Check sheet for the modelled part. Datum: model origin and axes. Units: mm. A direction names the side the tool comes from. Give positions to 0.01 mm unless a question says otherwise; leave off trailing zeros. Loops run counter-clockwise (first coordinate to the right, second up) from the corner with the lowest first, then second, coordinate; pieces in that order, holes last. Notation, with made-up numbers: (28.25, 76) - (76.25, 76) arc R30 ccw to (76.25, 108) - close; hole circle Ø2 at (-20, 7.25). An arc over 180 degrees is marked (long way). Answer in a Markdown table with one row per item. Add a question column.
(1) Sectioned sample at A-A on x = 5.5. Enter the section's corners in (y, z).
(2) Sectioned sample at B-B on y = 3. Enter the section's corners in (x, z).
(3) Sectioned sample at C-C on x = 13.5. Enter the section's corners in (y, z), then the cut area to 3 significant figures.
(4) Draft check along Z on faces 6 (the face through (5.57, 2.94, -4)), 7 (the face through (-5.5, 4.3, -4.6)), 8 (the face through (5.652, -0.74, -2.053)). Enter one of: released by +Z, released by -Z, zero draft, split by the parting line, or undercut.
(5) Sectioned sample at D-D on z = -10.25. Enter the section's corners in (x, y), then the cut area to 3 significant figures.
(6) Set-up check for faces 1 (the face through (5.4, 0, -1.9)), 2 (the face through (-6.355, 3.938, -7.763)), 3 (the face through (6.55, 6.74, -8.04)), 4 (the face through (17.345, 2.062, -7.763)), 5 (the face through (-2.7, 3.52, -4.2)): record each of +Z, -Z, +X, -X, +Y, -Y from which the full face is reachable in a straight line by a thin tool's end or side.
(7) Go/stop test with flat-tipped pins: P1, Ø3, axis at x = -4.5, y = 5.5, coming from the -Z side; P2, Ø4, axis at x = -1, y = 5.5, coming from the -Z side; P3, Ø2, axis at y = 5, z = -9.5, coming from the -X side. Record where each tip stops, or that it passes through.
(8) Thickness scan on L1, parallel to X at y = 1, z = -5.5; L2, parallel to X at y = 0.75, z = -5.5; L3, parallel to Y at x = 8, z = -3.25. Record the ranges inside material, lowest first.
from build123d import *

# Parameters (mm, degrees)
SKETCH1_W      = 11
SKETCH1_H      = 11
EXTRUDE1_DEPTH = 6
SKETCH2_R      = 1.4
EXTRUDE2_DEPTH = 5.5
EXTRUDE3_START = 5.5
SKETCH3_R      = 1.4
EXTRUDE3_DEPTH = 5.5
SKETCH4_R      = 2.75
EXTRUDE4_DEPTH = 1.5
SKETCH5_R      = 3.45
EXTRUDE5_DEPTH = 1.5
SKETCH6_R      = 2.45
EXTRUDE6_DEPTH = 1.7
EXTRUDE7_START = 1.7
SKETCH7_R      = 2.45
EXTRUDE7_DEPTH = 1.7
SKETCH8_R      = 1.5
EXTRUDE8_DEPTH = 24.091989953
FILLET1_R      = 5.5
FILLET3_R      = 0.5


with BuildPart() as part:
    # Sketch1 → Extrude1 (new body)
    with BuildSketch(Plane(origin=(0, 0, 0), x_dir=(1, 0, 0), z_dir=(0, 1, 0))):
        with Locations((5.5, 5.5)):
            Rectangle(SKETCH1_W, SKETCH1_H)
    extrude(amount=EXTRUDE1_DEPTH)

    # Sketch2 → Extrude2 (add)
    with BuildSketch(Plane(origin=(11, 0, 0), x_dir=(0, 0, -1), z_dir=(1, 0, 0))):
        with Locations(Location((5.5, 3, 0), (0, 0, 180))):
            Circle(SKETCH2_R)
    extrude(amount=EXTRUDE2_DEPTH)

    # Sketch3 → Extrude3 (add)
    with BuildSketch(Plane.ZY.offset(EXTRUDE3_START)):
        with Locations((-5.5, 3)):
            Circle(SKETCH3_R)
    extrude(amount=-EXTRUDE3_DEPTH)

    # Sketch4 → Extrude4 (add)
    with BuildSketch(Plane(origin=(0, 6, 0), x_dir=(1, 0, 0), z_dir=(0, 1, 0))):
        with Locations(Location((5.5, 5.5, 0), (0, 0, 90))):
            Circle(SKETCH4_R)
    extrude(amount=EXTRUDE4_DEPTH)

    # Sketch5 → Extrude5 (add)
    with BuildSketch(Plane.XZ):
        with Locations(Location((5.5, -5.5, 0), (0, 0, 270))):
            Circle(SKETCH5_R)
    extrude(amount=EXTRUDE5_DEPTH)

    # Sketch6 → Extrude6 (add)
    with BuildSketch(Plane(origin=(16.5, 0, 0), x_dir=(0, 0, -1), z_dir=(1, 0, 0))):
        with Locations((5.5, 3)):
            Circle(SKETCH6_R)
    extrude(amount=EXTRUDE6_DEPTH)

    # Sketch7 → Extrude7 (add)
    with BuildSketch(Plane.ZY.offset(5.5).offset(EXTRUDE7_START)):
        with Locations(Location((-5.5, 3, 0), (0, 0, 180))):
            Circle(SKETCH7_R)
    extrude(amount=-EXTRUDE7_DEPTH)

    # Sketch8 → Extrude8 (cut, through all)
    with BuildSketch(Plane.XZ.offset(1.5)):
        with Locations(Location((5.5, -5.5, 0), (0, 0, 270))):
            Circle(SKETCH8_R)
    extrude(amount=-EXTRUDE8_DEPTH, mode=Mode.SUBTRACT)

    # Fillet1
    # the kernel refuses this fillet: 5.5 mm, written as the material it takes off along each edge
    with BuildSketch(Plane(origin=(0, -13.75, 0), x_dir=(0, 0, -1), z_dir=(0, 1, 0))) as fillet1_piece_1_section:
        with BuildLine():
            CenterArc((FILLET1_R, -FILLET1_R), FILLET1_R, 90, 90)
            Line((0, -FILLET1_R), (0, 0))
            Line((0, 0), (FILLET1_R, 0))
        make_face()
    fillet1_piece_1 = extrude(amount=33.5, mode=Mode.PRIVATE)
    fillet1_piece_1 = fillet1_piece_1 - Plane(origin=(1.247523626, 3, -5.5), x_dir=(0, 0, 1), z_dir=(-1, 0, 0)) * Cylinder(1.4, 89, mode=Mode.PRIVATE)
    with BuildSketch(Plane(origin=(0, -13.75, -11), x_dir=(0, 0, 1), z_dir=(0, 1, 0))) as fillet1_piece_2_section:
        with BuildLine():
            CenterArc((FILLET1_R, FILLET1_R), FILLET1_R, 180, 90)
            Line((0, FILLET1_R), (0, 0))
            Line((0, 0), (FILLET1_R, 0))
        make_face()
    fillet1_piece_2 = extrude(amount=33.5, mode=Mode.PRIVATE)
    fillet1_piece_2 = fillet1_piece_2 - Plane(origin=(1.247523509, 3, -5.5), x_dir=(0, 0, 1), z_dir=(-1, 0, 0)) * Cylinder(1.4, 89, mode=Mode.PRIVATE)
    with BuildSketch(Plane(origin=(11, -13.75, -11), x_dir=(-1, 0, 0), z_dir=(0, 1, 0))) as fillet1_piece_3_section:
        with BuildLine():
            CenterArc((FILLET1_R, FILLET1_R), FILLET1_R, 180, 90)
            Line((0, FILLET1_R), (0, 0))
            Line((0, 0), (FILLET1_R, 0))
        make_face()
    fillet1_piece_3 = extrude(amount=33.5, mode=Mode.PRIVATE)
    fillet1_piece_3 = fillet1_piece_3 - Plane(origin=(9.752477266, 3, -5.5), x_dir=(0, 0, 1), z_dir=(-1, 0, 0)) * Cylinder(1.4, 89, mode=Mode.PRIVATE)
    with BuildSketch(Plane(origin=(11, -13.75, 0), x_dir=(-1, 0, 0), z_dir=(0, 1, 0))) as fillet1_piece_4_section:
        with BuildLine():
            CenterArc((FILLET1_R, -FILLET1_R), FILLET1_R, 90, 90)
            Line((0, -FILLET1_R), (0, 0))
            Line((0, 0), (FILLET1_R, 0))
        make_face()
    fillet1_piece_4 = extrude(amount=33.5, mode=Mode.PRIVATE)
    fillet1_piece_4 = fillet1_piece_4 - Plane(origin=(9.752475868, 3, -5.5), x_dir=(0, 0, 1), z_dir=(-1, 0, 0)) * Cylinder(1.4, 89, mode=Mode.PRIVATE)
    add([fillet1_piece_1, fillet1_piece_2, fillet1_piece_3, fillet1_piece_4], mode=Mode.SUBTRACT)

    # Fillet3
    fillet3_edges = [part.edges().sort_by_distance(p)[0] for p in [
        (16.5, 3, -3.05),
        (18.2, 3, -3.05),
        (-5.5, 3, -3.05),
        (-7.2, 3, -3.05),
    ]]
    fillet(fillet3_edges, radius=FILLET3_R)


solid = part.part
Reply:
| question | item | result |
|---|---|---|
| 1 | outline | (-1.5, -8.95) - (0, -8.95) - (0, -11) - (6, -11) - (6, -8.25) - (7.5, -8.25) - (7.5, -7) - (-1.5, -7) - close; (-1.5, -4) - (7.5, -4) - (7.5, -2.75) - (6, -2.75) - (6, 0) - (0, 0) - (0, -2.05) - (-1.5, -2.05) - close |
| 2 | outline | (-7.2, -7.45) arc R0.5 ccw to (-6.7, -7.95) - (-6, -7.95) arc R0.5 ccw to (-5.5, -7.45) - (-5.5, -6.9) - (0.18, -6.9) arc R5.5 ccw to (10.82, -6.9) - (16.5, -6.9) - (16.5, -7.45) arc R0.5 ccw to (17, -7.95) - (17.7, -7.95) arc R0.5 ccw to (18.2, -7.45) - (18.2, -3.55) arc R0.5 ccw to (17.7, -3.05) - (17, -3.05) arc R0.5 ccw to (16.5, -3.55) - (16.5, -4.1) - (10.82, -4.1) arc R5.5 ccw to (0.18, -4.1) - (-5.5, -4.1) - (-5.5, -3.55) arc R0.5 ccw to (-6, -3.05) - (-6.7, -3.05) arc R0.5 ccw to (-7.2, -3.55) - close; hole circle Ø3 at (5.5, -5.5) |
| 3 | outline | circle Ø2.8 at (3, -5.5) |
| 3 | area | 6.16 mm^2 |
| 4 | face 6 | undercut |
| 4 | face 7 | zero draft |
| 4 | face 8 | split by the parting line |
| 5 | outline | (2.73, 0) - (8.27, 0) - (8.27, 6) - (2.73, 6) - close |
| 5 | area | 33.3 mm^2 |
| 6 | face 1 | -Y |
| 6 | face 2 | -X |
| 6 | face 3 | +Y |
| 6 | face 4 | +X |
| 6 | face 5 | none |
| 7 | P1 | z = -7.22 |
| 7 | P2 | z = -8.66 |
| 7 | P3 | x = 0.89 |
| 8 | L1 | -7.2 to -5.5, 0 to 4, 7 to 11, 16.5 to 18.2 |
| 8 | L2 | -7.1 to -5.6, 0 to 4, 7 to 11, 16.6 to 18.1 |
| 8 | L3 | -1.5 to 6 |
